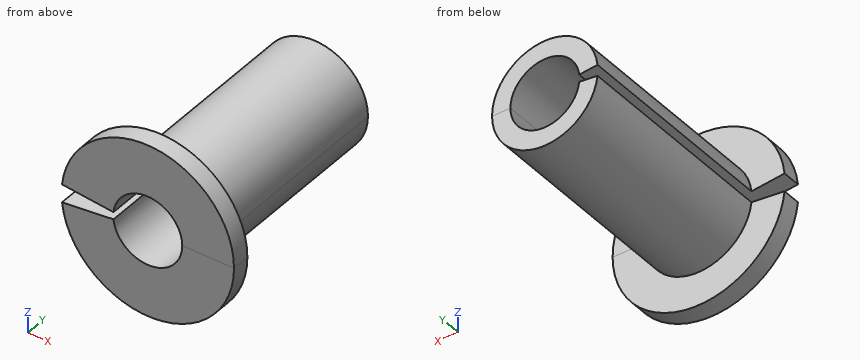
from build123d import *
from build123d.topology import SkipClean

# Parameters (mm, degrees)
REVOLVE1_ANGLE = 348


with BuildPart() as part:
    # Sketch1 → Revolve1 (revolve, symmetric)
    with SkipClean():  # the faces are left unmerged after this step: merging them gives an invalid solid
        with BuildSketch(Plane.XY) as revolve1_sk:
            Polygon((3, 20), (3, 0), (7.5, 0), (7.5, 1.6), (4.6, 1.6), (4.6, 20), align=None)
        revolve(axis=Axis((0, 0, 0), (0, 1, 0)), revolution_arc=REVOLVE1_ANGLE / 2)
        revolve(revolve1_sk.sketch, axis=Axis((0, 0, 0), (0, -1, 0)), revolution_arc=REVOLVE1_ANGLE / 2)
    add(part.part.scale(1), mode=Mode.REPLACE)  # the faces are merged on a copy


solid = part.part
For this review, take the finished solid that the model builds, in its own axes (mm). Round coordinates to 2 decimals unless told otherwise and drop trailing zeros. Order: outer loops, then holes, each group sorted by start corner. A loop starts at its lowest first (then second) coordinate and runs counter-clockwise, first axis right, second up. Notation, with made-up numbers: (10, 21) -> (39, 21) arc R34 cw to (39, 55) -> close; hole circle Ø9 at (-20.75, 12). An arc over 180 degrees is marked (long way). Write item = value, one per line. Start each with the question number.
1) Take a section at A-A on x = 0. State the section outline as (y, z) points, plus the area to 3 significant figures.
2) Insertion check: pin 1 (3 mm diameter, centred on x = -3.5, y = 17.5, fed in from +Z); pin 2 (1.5 mm diameter, centred on y = 8, z = -4, fed in from -X); pin 3 (5 mm diameter, centred on x = 6, z = 5, fed in from +Y). Each pin has a flat end and moves straight along its axis. Give the tip position at first contact, or say it passes through.
3) Take a section at B-B on z = -3.5. State the section outline as (x, y) points.
4) To check wall thickness, follow line 1 (Y direction, x = 4.5, z = 3.5); line 2 (Z direction, x = -0.75, y = 6.25); line 3 (Z direction, x = 0.5, y = 3). State the ranges of each line that lie inside material, in increasing order. Write a range as from..to.
5) Take a section at C-C on x = -2.75. State the section outline as (y, z) points.
6) Take a section at D-D on y = 7.5. State the section outline as (x, z) points, plus the area to 3 significant figures.
Verdict:
q1.outline = (0, -7.5) -> (1.6, -7.5) -> (1.6, -4.6) -> (20, -4.6) -> (20, -3) -> (0, -3) -> close; (0, 3) -> (20, 3) -> (20, 4.6) -> (1.6, 4.6) -> (1.6, 7.5) -> (0, 7.5) -> close
q1.area = 73.3 mm2
q2.pin_1 = 4.14
q2.pin_2 = -3.26
q2.pin_3 = 1.6
q3.outline = (-6.63, 0) -> (6.63, 0) -> (6.63, 1.6) -> (2.98, 1.6) -> (2.98, 20) -> (-2.98, 20) -> (-2.98, 1.6) -> (-6.63, 1.6) -> close
q4.line_1 = 0..1.6
q4.line_2 = -4.54..-2.9, 2.9..4.54
q4.line_3 = -4.57..-2.96, 2.96..4.57
q5.outline = (0, -6.98) -> (1.6, -6.98) -> (1.6, -3.69) -> (20, -3.69) -> (20, -1.2) -> (0, -1.2) -> close; (0, 1.2) -> (20, 1.2) -> (20, 3.69) -> (1.6, 3.69) -> (1.6, 6.98) -> (0, 6.98) -> close
q6.outline = (-4.57, -0.48) arc R4.6 ccw (long way) to (-4.57, 0.48) -> (-2.98, 0.31) arc R3 cw (long way) to (-2.98, -0.31) -> close
q6.area = 36.9 mm2
